Geometry: see drawing. Coordinates: mm, zero at the bounding-box minimum. Give positions to 0.01 mm unless a question says otherwise; leave off trailing zeros. Order: outer loops, then holes, each group sorted by start corner. A loop starts at its lowest first (then second) coordinate and runs counter-clockwise, first axis right, second up. Notation, with made-up numbers: (2.25, 74.25) - (56.25, 74.25) arc R22 cw to (56.25, 95.25) - close; hole circle Ø3 at (-9, 60.5). An arc over 180 degrees is marked (long way). Write item = value, one per line. Start each with the question number.
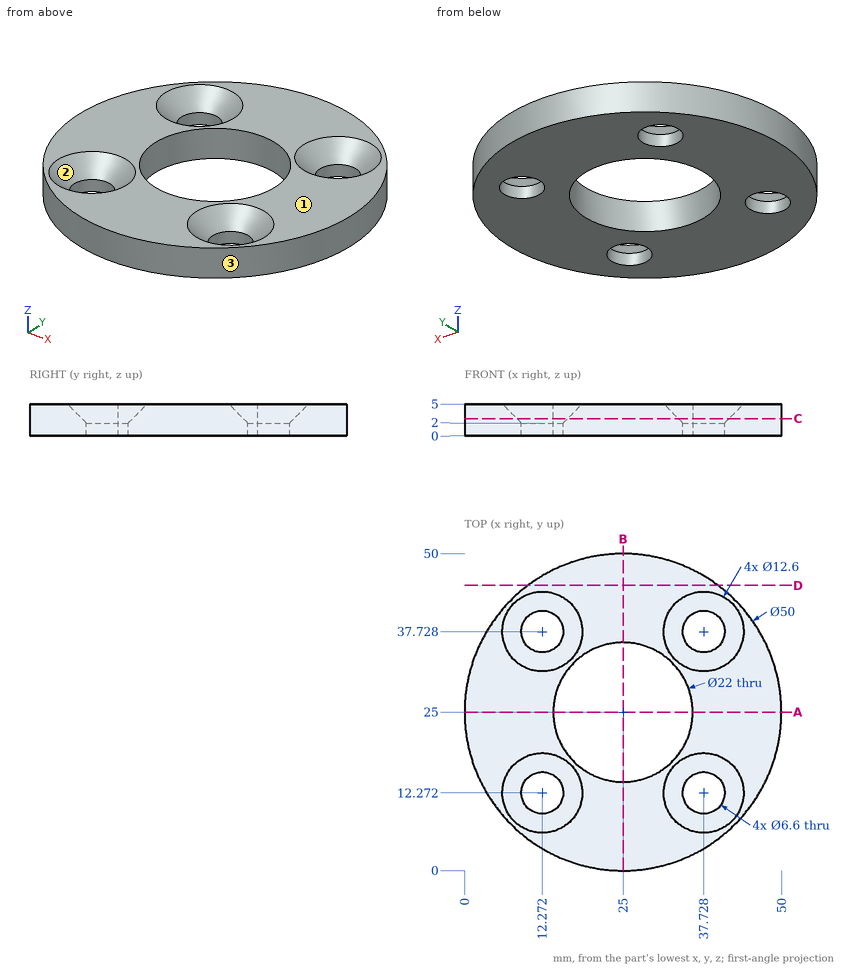
Q1. Contact query for flat-ended pins moving along their axis: pin 1 (7.5 mm diameter, centred on x = 12.27, y = 12.27, fed in from +Z); pin 2 (3 mm diameter, centred on y = 19, z = 0.5, fed in from +X); pin 3 (1.5 mm diameter, centred on x = 24.5, z = 3, fed in from -Y). Output: stop coordinate, or through.
Q2. Material intervals for line 1 along X through (y, z) = (12.5, 4.2); line 2 along X through (y, z) = (40.5, 2.75) (1 decimal); line 3 along X through (y, z) = (16, 4.25) (1 decimal), sorted ascending. Write a range as from..to.
Q3. Section C-C, the plane z = 2.7. Return the cut outline in (x, y).
Q4. Section D-D, the plane y = 45. Return the cut outline in (x, z), then the cut area to 3 significant figures.
Q5. Section A-A, the plane y = 25. Return the cut outline in (x, z).
Q6. Pull-direction query (X, two-part tool) for the marked faces 1, 2 and 3; classes: +X half, -X half, draft (parallel to the pull), parting line (faces both ways), or undercut.
The answers:
q1.pin_1 = 2.45
q1.pin_2 = 49.59
q1.pin_3 = 0
q2.line_1 = 3.35..6.78, 17.77..32.23, 43.22..46.65
q2.line_2 = 5.4..9.3, 15.2..34.8, 40.7..44.6
q2.line_3 = 1.7..8.2, 16.4..18.7, 31.3..33.6, 41.8..48.3
q3.outline = circle Ø50 at (25, 25); hole circle Ø8 at (12.27, 12.27); hole circle Ø8 at (12.27, 37.73); hole circle Ø22 at (25, 25); hole circle Ø8 at (37.73, 12.27); hole circle Ø8 at (37.73, 37.73)
q4.outline = (10, 0) - (40, 0) - (40, 5) - (10, 5) - close
q4.area = 150 mm²
q5.outline = (0, 0) - (14, 0) - (14, 5) - (0, 5) - close; (36, 0) - (50, 0) - (50, 5) - (36, 5) - close
q6.face_1 = draft
q6.face_2 = undercut
q6.face_3 = parting line
